Autodesk Inventor part; units mm, degrees
ref_plane "YZ Plane" through (0, 0, 0) normal (1, 0, 0) x (0, 1, 0)
ref_plane "XZ Plane" through (0, 0, 0) normal (0, 1, 0) x (-1, 0, 0)
ref_plane "XY Plane" through (0, 0, 0) normal (0, 0, 1) x (1, 0, 0)
sketch "스케치4" plane through (0, 0, 0) normal (0, 1, 0) x (-1, 0, 0)
  line L0 (-2, 5.5) -> (-2, -5.5)
  line L1 (-2, -5.5) -> (2, -5.5)
  line L2 (2, -5.5) -> (2, 5.5)
  line L3 (2, 5.5) -> (-2, 5.5)
  line L4 (-2, 5.5) -> (2, -5.5) construction
  line L5 (-2, -5.5) -> (2, 5.5) construction
  line L6 (15.7602, 19.8) -> (-23.0581, 19.8) construction
  line L7 (-2, 34.1) -> (-2, 45.1)
  line L8 (-2, 45.1) -> (2, 45.1)
  line L9 (2, 45.1) -> (2, 34.1)
  line L10 (2, 34.1) -> (-2, 34.1)
  line L11 (-2, 34.1) -> (2, 45.1) construction
  line L12 (-2, 45.1) -> (2, 34.1) construction
  point P0 (0, 0)
  point P1 (0, 0)
  point P2 (0, 39.6)
  point P3 (0, 39.6)
  dimension "d12" = 11
  dimension "d13" = 4
  dimension "d42" = 19.8
extrude "돌출3" add sketch "스케치4" along normal blind 77
sketch "스케치5" plane through (0, 0, 0) normal (0, -1, 0) x (1, 0, 0)
  line L0 (-10.5, -5.5) -> (10.5, -5.5)
  line L1 (10.5, -5.5) -> (10.5, 5.5)
  line L2 (10.5, 5.5) -> (-10.5, 5.5)
  line L3 (-10.5, 5.5) -> (-10.5, -5.5)
  line L4 (-10.5, -5.5) -> (10.5, 5.5) construction
  line L5 (10.5, -5.5) -> (-10.5, 5.5) construction
  line L6 (0, 5.5) -> (0, -5.5) construction
  line L7 (10.5, 5.5) -> (12.5, 5.5)
  line L8 (12.5, 5.5) -> (12.5, -5.5)
  line L9 (12.5, -5.5) -> (10.5, -5.5)
  line L10 (-10.5, 5.5) -> (-12.5, 5.5)
  line L11 (-12.5, 5.5) -> (-12.5, -5.5)
  line L12 (-12.5, -5.5) -> (-10.5, -5.5)
  line L13 (-22.4262, 19.8) -> (40.7349, 19.8) construction
  line L14 (-10.5, 45.1) -> (10.5, 45.1)
  line L15 (10.5, 45.1) -> (10.5, 34.1)
  line L16 (10.5, 34.1) -> (-10.5, 34.1)
  line L17 (-10.5, 34.1) -> (-10.5, 45.1)
  line L18 (-10.5, 45.1) -> (10.5, 34.1) construction
  line L19 (10.5, 45.1) -> (-10.5, 34.1) construction
  line L20 (0, 34.1) -> (0, 45.1) construction
  line L21 (10.5, 34.1) -> (12.5, 34.1)
  line L22 (12.5, 34.1) -> (12.5, 45.1)
  line L23 (12.5, 45.1) -> (10.5, 45.1)
  line L24 (-10.5, 34.1) -> (-12.5, 34.1)
  line L25 (-12.5, 34.1) -> (-12.5, 45.1)
  line L26 (-12.5, 45.1) -> (-10.5, 45.1)
  point P0 (0, 0)
  point P1 (0, 0)
  point P2 (0, 39.6)
  point P3 (0, 39.6)
  dimension "d16" = 21
  dimension "d17" = 11
  dimension "d18" = 2
  dimension "d43" = 19.8
extrude "돌출4" add sketch "스케치5" along normal blind 2
extrude "돌출5" add sketch "스케치5" along normal blind 22 contours L12 L11 L10 L3 | L1 L7 L8 L9 | L17 L24 L25 L26 | L23 L22 L21 L15
sketch "스케치6" plane through (-12.5, 0, -5.5) normal (-1, 0, 0) x (0, 0, 1)
  line L0 (11, 0) -> (0, 0)
  line L1 (0, 0) -> (0, -22)
  line L2 (11, -22) -> (0, -22)
  line L3 (11, 0) -> (11, -22)
  circle A0 centre (5.5, -12) radius 1.5
  line L4 (25.3, -63.5481) -> (25.3, 115.0897)
  line L5 (11, 0) -> (11, 77)
  line L6 (39.6, -22) -> (50.6, -22)
  circle A1 centre (45.1, -12) radius 1.5
  point P0 (5.5, 0)
  point P1 (25.3, 25.7708)
  dimension "d23" = 3
  dimension "d24" = 10
  dimension "d44" = 14.3
extrude "돌출6" cut sketch "스케치6" against normal through all contours A0 | A1
sketch "스케치7" plane through (-2, 77, -5.5) normal (-1, 0, 0) x (0, 0, 1)
  line L0 (0, -77) -> (11, -77)
  line L1 (11, -77) -> (11, 0)
  line L2 (0, 0) -> (11, 0)
  line L3 (0, -77) -> (0, 0)
  line L4 (0, -73) -> (11, -73) construction
  line L5 (0, -4) -> (11, -4) construction
  line L6 (0, -69) -> (11, -69) construction
  circle A0 centre (5.5, -4) radius 1.5
  circle A1 centre (5.5, -69) radius 1.5
  line L7 (5.5, -69) -> (5.5, -4) construction
  circle A2 centre (5.5, -64) radius 1.5
  circle A3 centre (5.5, -59) radius 1.5
  circle A4 centre (5.5, -54) radius 1.5
  circle A5 centre (5.5, -49) radius 1.5
  circle A6 centre (5.5, -44) radius 1.5
  circle A7 centre (5.5, -39) radius 1.5
  circle A8 centre (5.5, -34) radius 1.5
  circle A9 centre (5.5, -29) radius 1.5
  circle A10 centre (5.5, -24) radius 1.5
  circle A11 centre (5.5, -19) radius 1.5
  circle A12 centre (5.5, -14) radius 1.5
  circle A13 centre (5.5, -9) radius 1.5
  line L8 (25.3, -134.2838) -> (25.3, 22.0863) construction
  line L9 (50.6, -77) -> (39.6, -77)
  line L10 (39.6, -77) -> (39.6, 0)
  line L11 (50.6, 0) -> (39.6, 0)
  line L12 (50.6, -77) -> (50.6, 0)
  line L13 (50.6, -73) -> (39.6, -73) construction
  line L14 (50.6, -4) -> (39.6, -4) construction
  line L15 (50.6, -69) -> (39.6, -69) construction
  circle A14 centre (45.1, -4) radius 1.5
  circle A15 centre (45.1, -69) radius 1.5
  line L16 (45.1, -69) -> (45.1, -4) construction
  circle A16 centre (45.1, -64) radius 1.5
  circle A17 centre (45.1, -59) radius 1.5
  circle A18 centre (45.1, -54) radius 1.5
  circle A19 centre (45.1, -49) radius 1.5
  circle A20 centre (45.1, -44) radius 1.5
  circle A21 centre (45.1, -39) radius 1.5
  circle A22 centre (45.1, -34) radius 1.5
  circle A23 centre (45.1, -29) radius 1.5
  circle A24 centre (45.1, -24) radius 1.5
  circle A25 centre (45.1, -19) radius 1.5
  circle A26 centre (45.1, -14) radius 1.5
  circle A27 centre (45.1, -9) radius 1.5
  point P0 (5.5, -77)
  point P1 (45.1, -77)
  dimension "d27" = 4
  dimension "d28" = 4
  dimension "d29" = 4
  dimension "d30" = 3
  dimension "d31" = 5.5
  dimension "d32" = 3
  dimension "d35" = 5
  dimension "d45" = 14.3
extrude "돌출7" cut sketch "스케치7" against normal through all contours A0 | A1 | A2 | A3 | A4 | A5 | A6 | A7 | A8 | A9 | A10 | A11 | A12 | A13 | A14 | A15 | A16 | A17 | A18 | A19 | A20 | A21 | A22 | A23 | A24 | A25 | A26 | A27
sketch "스케치9" plane through (2, 77, 34.1) normal (0, 0, -1) x (-1, 0, 0)
  line L0 (-8.5, -79) -> (-8.5, -77)
  line L1 (-10.5, -77) -> (0, -77)
  line L2 (-8.5, -79) -> (12.5, -79)
  line L3 (12.5, -79) -> (12.5, -77)
  line L4 (14.5, -77) -> (4, -77)
  line L5 (14.5, -77) -> (4, -77)
  line L6 (4, -77) -> (4, 0)
  line L7 (0, 0) -> (4, 0)
  line L8 (0, -77) -> (0, 0)
  line L9 (0, -77) -> (-10.5, -77)
  line L10 (-10.5, -77) -> (-10.5, -99)
  line L11 (-8.5, -99) -> (-10.5, -99)
  line L12 (-8.5, -79) -> (-8.5, -99)
  line L13 (12.5, -79) -> (-8.5, -79)
  line L14 (12.5, -79) -> (12.5, -99)
  line L15 (14.5, -99) -> (12.5, -99)
  line L16 (14.5, -77) -> (14.5, -99)
  line L17 (0, -77) -> (4, -77)
  point P0 (2, -77)
  point P1 (4, -77)
extrude "돌출8" add sketch "스케치9" along normal up to surface (28.6 mm away) contours L0 L1 L17 L4 L3 L2
properties part number "catcher_2ea"
Can you work these out from the model? Positions are in its coordinate system, mm. A direction names the side the tool comes from. Round coordinates to 2 decimals unless told otherwise and drop trailing zeros. Loops run counter-clockwise (first coordinate to the right, second up) from the corner with the lowest first, then second, coordinate; pieces in that order, holes last. Notation, with made-up numbers: M 31,19.25 L 75,19.25 A32 ccw 75,48.25 Z; hole C 11,-38 d11. An arc over 180 degrees is marked long. Write item = value, one per line. Start each with the question number.
(1) Suppose I cut it at C-C on y = 70.5. Write out the boundary of the cut face in (x, z), plus the area to 3 significant figures.
(2) Suppose I cut it at B-B on y = 53. Write out the boundary of the cut face in (x, z), plus the area to 3 significant figures.
(3) Which directions (+Z, -Z, +X, -X, +Y, -Y) give clear straight access to the entire face, cutting with the end or side of a thin tool? Please do faces 5 (the face through (-12, -22, 0)), 6 (the face through (2, 38, 37)), 7 (the face through (-10.5, -1, 20)), 8 (the face through (-10.5, -14, 0)).
(4) I need wall thicknesses on line 1 along Z through (x, y) = (-0.5, 68); line 2 along Y through (x, z) = (8.5, 12); line 3 along X through (y, z) = (-3, 43). Which ranges of each line are inside material? Lowest first, please.
(5) Suppose I cut it at A-A on y = -12. Give the number of separate pieces and of enclosed holes in the cut face, plus the area to 3 significant figures.
(6) If we mould it in two halves opening along Y, with no side actions, what happens to faces 1 (the face through (-0.03, 13.07, 38.1)), 2 (the face through (0, 77, 0)), 3 (the face through (2, 38, 3)), 4 (the face through (-0.03, 19.01, 38.49))? For each: released by +Y, released by -Y, zero draft, split by the parting line, or undercut.
(7) I'm going to push flat-ended pins straight in: P1, Ø5.5, axis at y = 57.5, z = -1, coming from the -X side; P2, Ø1, axis at y = -0.5, z = 26.5, coming from the +X side; P3, Ø10, axis at y = 20.5, z = 0, coming from the +X side; P4, Ø10, axis at x = -9, y = 58.5, coming from the -Z side. Where does each tip first touch, or does it pass through?
Answer block:
q1.outline = M -2,-5.5 L 2,-5.5 L 2,5.5 L -2,5.5 Z; M -2,34.1 L 2,34.1 L 2,45.1 L -2,45.1 Z
q1.area = 88.0 mm²
q2.outline = M -2,-5.5 L 2,-5.5 L 2,-1.5 L -2,-1.5 Z; M -2,1.5 L 2,1.5 L 2,5.5 L -2,5.5 Z; M -2,34.1 L 2,34.1 L 2,38.1 L -2,38.1 Z; M -2,41.1 L 2,41.1 L 2,45.1 L -2,45.1 Z
q2.area = 64.0 mm²
q3.face_5 = +Z, -Z, +X, -X, -Y
q3.face_6 = +Z, -Z, +X, +Y
q3.face_7 = -X, +Y, -Y
q3.face_8 = +Z, -Z, -Y
q4.line_1 = -5.5 to -1.5, 1.5 to 5.5, 34.1 to 38.1, 41.1 to 45.1
q4.line_2 = -2 to 0
q4.line_3 = -12.5 to -10.5, 10.5 to 12.5
q5.separate_pieces = 8
q5.enclosed_holes = 0
q5.area = 64.0 mm²
q6.face_1 = undercut
q6.face_2 = released by +Y
q6.face_3 = zero draft
q6.face_4 = undercut
q7.P1 = -2
q7.P2 = 10.5
q7.P3 = 2
q7.P4 = through
